Work out the finished part from the listing and answer in its coordinate system (mm). A direction names the side the tool comes from. Round coordinates to 2 decimals unless told otherwise and drop trailing zeros. Write each loop counter-clockwise with the first axis right and the second up, starting at its lowest first coordinate (ties: lowest second). Pieces come first, ordered by that corner, then holes.
1. Find section D-D (x = 12). Write down the section's boundary in (y, z), and give its area (3 significant figures).
2. Straight lines are drawn through the part: probe 1 along X at (y, z) = (3.5, -11); probe 2 along Y at (x, z) = (-20.05, -32); probe 3 along Y at (x, z) = (-12, -12.5). For each, find the intervals that lie inside material, in ascending order.
3. Determine the mould class of faces 4 (the face through (-16.453, 16, -3)), 5 (the face through (-12.14, 14.07, -30.5)), 6 (the face through (31, 9.76, 2.46)) for opening direction X: pulls with the +X half, pulls with the -X half, needs draft (parallel to the pull), parting line crosses it, or undercut.
4. A tool of negligible diameter and unlimited length cuts with its end or side. For faces 1 (the face through (8, 4, -23)), 2 (the face through (-12, 21, -4)), 3 (the face through (-12, 14, -29.5)), from which of +Z, -Z, +X, -X, +Y, -Y can it reach the whole face along a straight path? Write none if from no direction.
5. Find section C-C (z = -23.5). Write down the section's boundary in (x, y).
6. Find section B-B (y = 10). Write down the section's boundary in (x, z).
7. Flat-ended cylindrical pins translate along their axes: pin 1 Ø24 at (x, z) = (-7, -17.5) entering from -Y; pin 2 Ø2 at (x, y) = (-18, 8.5) entering from -Z; pin 3 Ø2 at (x, z) = (-11, -16.5) entering from +Y; pin 4 Ø1.8 at (y, z) = (14, -4) entering from -X. Find the tip coordinate at first contact, or state that the pin passes through.
8. Find section A-A (x = 0). Write down the section's boundary in (y, z), and give its area (3 significant figures).
```python
from build123d import *

# Parameters (mm, degrees)
CROQUIS1_R               = 32.5
CROQUIS1_R_2             = 8.5
SALIENTE_EXTRUIR1_DEPTH  = 5
CROQUIS3_W               = 30
CROQUIS3_H               = 10
SALIENTE_EXTRUIR5_DEPTH  = 50
CROQUIS4_W               = 7
CROQUIS4_H               = 50
SALIENTE_EXTRUIR6_DEPTH  = 5
CROQUIS5_W               = 25
CROQUIS5_H               = 35
SALIENTE_EXTRUIR7_DEPTH  = 6
CROQUIS6_W               = 8.5
CROQUIS6_H               = 5.5
CROQUIS6_W_2             = 2
CROQUIS6_H_2             = 7
SALIENTE_EXTRUIR8_DEPTH  = 13
CROQUIS7_R               = 1.5
CORTAR_EXTRUIR1_DEPTH    = 20
CROQUIS8_W               = 16
CROQUIS8_H               = 5
SALIENTE_EXTRUIR9_DEPTH  = 5
SALIENTE_EXTRUIR10_DEPTH = 10
CROQUIS11_R              = 1
CORTAR_EXTRUIR2_DEPTH    = 5
CROQUIS13_R              = 1.5
CORTAR_EXTRUIR3_DEPTH    = 10


with BuildPart() as part:
    # Croquis1 → Saliente-Extruir1 (new body)
    with BuildSketch(Plane.XY):
        Circle(CROQUIS1_R)
        Circle(CROQUIS1_R_2, mode=Mode.SUBTRACT)
    extrude(amount=SALIENTE_EXTRUIR1_DEPTH)

    # Croquis3 → Saliente-Extruir5 (add)
    with BuildSketch(Plane(origin=(0, 0, 0), x_dir=(-1, 0, 0), z_dir=(0, 0, -1))):
        with Locations((0, -8)):
            Rectangle(CROQUIS3_W, CROQUIS3_H)
    extrude(amount=SALIENTE_EXTRUIR5_DEPTH)

    # Croquis4 → Saliente-Extruir6 (add)
    with BuildSketch(Plane(origin=(0, -3, 0), x_dir=(1, 0, 0), z_dir=(0, 1, 0))):
        with Locations((-11.5, 25)):
            Rectangle(CROQUIS4_W, CROQUIS4_H)
        with Locations((11.5, 25)):
            Rectangle(CROQUIS4_W, CROQUIS4_H)
    extrude(amount=SALIENTE_EXTRUIR6_DEPTH)

    # Croquis5 → Saliente-Extruir7 (add)
    with BuildSketch(Plane(origin=(0, 2, 0), x_dir=(1, 0, 0), z_dir=(0, 1, 0))):
        with Locations((-20.45298686, 17.5)):
            Rectangle(CROQUIS5_W, CROQUIS5_H)
    extrude(amount=SALIENTE_EXTRUIR7_DEPTH)

    # Croquis6 → Saliente-Extruir8 (add)
    with BuildSketch(Plane(origin=(0, 8, 0), x_dir=(1, 0, 0), z_dir=(0, 1, 0))):
        with Locations((-12.20298686, 32.25)):
            Rectangle(CROQUIS6_W, CROQUIS6_H)
        with Locations((-20.45298686, 32.25)):
            Rectangle(CROQUIS6_W_2, CROQUIS6_H)
        with Locations((-12.20298686, 3.5)):
            Rectangle(CROQUIS6_W, CROQUIS6_H_2)
        with Locations((-20.45298686, 3.5)):
            Rectangle(CROQUIS6_W_2, CROQUIS6_H_2)
    extrude(amount=SALIENTE_EXTRUIR8_DEPTH)

    # Croquis7 → Cortar-Extruir1 (cut)
    with BuildSketch(Plane(origin=(-7.95298686, 0, 0), x_dir=(0, 0, -1), z_dir=(1, 0, 0))):
        with Locations((32, 14)):
            Circle(CROQUIS7_R)
        with Locations((4, 14)):
            Circle(CROQUIS7_R)
    extrude(amount=-CORTAR_EXTRUIR1_DEPTH, mode=Mode.SUBTRACT)

    # Croquis8 → Saliente-Extruir9 (add)
    with BuildSketch(Plane(origin=(0, -3, 0), x_dir=(1, 0, 0), z_dir=(0, 1, 0))):
        with Locations((0, 47.5)):
            Rectangle(CROQUIS8_W, CROQUIS8_H)
    extrude(amount=SALIENTE_EXTRUIR9_DEPTH)

    # Croquis10 → Saliente-Extruir10 (add)
    with BuildSketch(Plane(origin=(0, 2, 0), x_dir=(1, 0, 0), z_dir=(0, 1, 0))):
        Polygon((8, 0), (15, 0), (15, 50), (-15, 50), (-15, 35), (-8, 35), (-8, 45), (8, 45), align=None)
    extrude(amount=SALIENTE_EXTRUIR10_DEPTH)

    # Croquis11 → Cortar-Extruir2 (cut)
    with BuildSketch(Plane(origin=(0, 0, -50), x_dir=(-1, 0, 0), z_dir=(0, 0, -1))):
        with Locations((-4, 0)):
            Circle(CROQUIS11_R)
        with Locations((-12, 0)):
            Circle(CROQUIS11_R)
        with Locations((4, 0)):
            Circle(CROQUIS11_R)
        with Locations((12, 0)):
            Circle(CROQUIS11_R)
    extrude(amount=-CORTAR_EXTRUIR2_DEPTH, mode=Mode.SUBTRACT)

    # Croquis13 → Cortar-Extruir3 (cut)
    with BuildSketch(Plane(origin=(0, 0, -50), x_dir=(-1, 0, 0), z_dir=(0, 0, -1))):
        Circle(CROQUIS13_R)
    extrude(amount=-CORTAR_EXTRUIR3_DEPTH, mode=Mode.SUBTRACT)


solid = part.part
```
Worked answers:
1. outline: (-30.2, 0) - (-13, 0) - (-13, -50) - (-1, -50) - (-1, -45) - (1, -45) - (1, -50) - (12, -50) - (12, 0) - (30.2, 0) - (30.2, 5) - (-30.2, 5) - close
1. area: 1,540 mm2
2. probe 1: x = -32.95 to -7.95, 8 to 15
2. probe 2: y = 2 to 12.5, 15.5 to 21
2. probe 3: y = -13 to 8
3. face 4: undercut
3. face 5: needs draft
3. face 6: parting line crosses it
4. face 1: +Y
4. face 2: -Z, +X, -X, +Y
4. face 3: -X, +Y
5. outline: (-32.95, 2) - (-15, 2) - (-15, -13) - (15, -13) - (15, 12) - (8, 12) - (8, -3) - (-8, -3) - (-8, 2) - (-7.95, 2) - (-7.95, 8) - (-32.95, 8) - close
6. outline: (-30.92, 0) - (-21.45, 0) - (-21.45, -7) - (-19.45, -7) - (-19.45, 0) - (-16.45, 0) - (-16.45, -7) - (-7.95, -7) - (-7.95, 0) - (8, 0) - (8, -45) - (-8, -45) - (-8, -35) - (-7.95, -35) - (-7.95, -29.5) - (-16.45, -29.5) - (-16.45, -35) - (-15, -35) - (-15, -50) - (15, -50) - (15, 0) - (30.92, 0) - (30.92, 5) - (-30.92, 5) - close; (-21.45, -35) - (-19.45, -35) - (-19.45, -29.5) - (-21.45, -29.5) - close
7. pin 1: stops at y = -13
7. pin 2: stops at z = -35
7. pin 3: stops at y = 8
7. pin 4: passes through
8. outline: (-32.5, 0) - (-13, 0) - (-13, -50) - (-1.5, -50) - (-1.5, -45) - (-3, -45) - (-3, 0) - (-8.5, 0) - (-8.5, 5) - (-32.5, 5) - close; (1.5, -50) - (12, -50) - (12, -45) - (1.5, -45) - close; (8.5, 0) - (32.5, 0) - (32.5, 5) - (8.5, 5) - close
8. area: 800 mm2
